Read the model definition and answer for the solid it produces. Units are mm, in the model's axes. A direction names the side the tool comes from. Coordinates: 2 decimals unless noted, no trailing zeros. Write each loop counter-clockwise with the first axis right and the second up, starting at its lowest first coordinate (ties: lowest second). Pieces come first, ordered by that corner, then holes. Notation, with made-up numbers: (50.25, 36) -> (101.25, 36) arc R5 ccw to (101.25, 41) -> close; hole circle Ø1 at (81.5, 67). An arc over 180 degrees is marked (long way). One line per item, written item: value. Start each with the question number.
from build123d import *

# Parameters (mm, degrees)
BOSS_EXTRUDE1_DEPTH          = 6.604
SKETCH2_R                    = 3.175
BOSS_EXTRUDE2_DEPTH          = 4.572
SKETCH3_R                    = 1.7907
CUT_EXTRUDE1_DEPTH           = 30.055416707
SKETCH4_R                    = 2.0193
CUT_EXTRUDE2_DEPTH           = 26.214451888
CUT_EXTRUDE2_DRAFT           = -4
CUT_EXTRUDE2_PROFILE_2_DEPTH = 26.214451888
CUT_EXTRUDE2_PROFILE_2_DRAFT = -4
SKETCH5_R                    = 1.7907
CUT_EXTRUDE3_DEPTH           = 6.604
SKETCH6_R                    = 2.0193
CUT_EXTRUDE4_DEPTH           = 6.604
CUT_EXTRUDE4_DRAFT           = -4
CUT_EXTRUDE4_PROFILE_2_DEPTH = 6.604
CUT_EXTRUDE4_PROFILE_2_DRAFT = -4


with BuildPart() as part:
    # Sketch1 → Boss-Extrude1 (new body)
    with BuildSketch(Plane.XY):
        Polygon((-11.5, -6.25), (-11.5, 6.25), (11.5, 6.25), (11.5, -6.25), (11.5, -9.498), (19.05, -9.498), (19.05, -6.25), (19.05, 10.822), (-19.05, 10.822), (-19.05, -6.25), (-19.05, -9.498), (-11.5, -9.498), align=None)
    extrude(amount=BOSS_EXTRUDE1_DEPTH)

    # Sketch2 → Boss-Extrude2 (add)
    with BuildSketch(Plane(origin=(0, 10.822, 0), x_dir=(1, 0, 0), z_dir=(0, 1, 0))):
        with BuildLine():
            Line((2.08, -11.464), (2.08, -6.604))
            Line((2.08, -6.604), (17.32, -6.604))
            Line((17.32, -6.604), (17.32, -11.464))
            ThreePointArc((17.32, -11.464), (9.7, -19.084), (2.08, -11.464))
        make_face()
        with Locations(Location((9.7, -11.464, 0), (0, 0, 180))):
            Circle(SKETCH2_R, mode=Mode.SUBTRACT)
    extrude(amount=-BOSS_EXTRUDE2_DEPTH)

    # Sketch3 → Cut-Extrude1 (cut, through all)
    with BuildSketch(Plane(origin=(0, 0, 0), x_dir=(-1, 0, 0), z_dir=(0, 0, -1))):
        with Locations((13.9, 0)):
            Circle(SKETCH3_R)
        with Locations((-13.9, 0)):
            Circle(SKETCH3_R)
    extrude(amount=-CUT_EXTRUDE1_DEPTH, mode=Mode.SUBTRACT)


with BuildPart() as cut_extrude2_tool:
    # Sketch4 → Cut-Extrude2 (with draft: the straight prism first)
    with BuildSketch(Plane.XY.offset(6.604)):
        with Locations((-13.9, 0)):
            Circle(SKETCH4_R)
    extrude(amount=-CUT_EXTRUDE2_DEPTH)
    # Cut-Extrude2: the draft: its side faces are tilted about the plane it starts from
    cut_extrude2_sides = [cut_extrude2_tool.faces().sort_by_distance(p)[0] for p in [
        (-15.9193, 0, -6.503225944),
    ]]
    draft(cut_extrude2_sides, Plane.XY.offset(6.604), CUT_EXTRUDE2_DRAFT)


with BuildPart() as part_1:
    add(part.part)

    # Cut-Extrude2: cut by cut_extrude2_tool
    add(cut_extrude2_tool.part, mode=Mode.SUBTRACT)


with BuildPart() as cut_extrude2_profile_2_tool:
    # Sketch4 → Cut-Extrude2 profile 2 (with draft: the straight prism first)
    with BuildSketch(Plane.XY.offset(6.604)):
        with Locations((13.9, 0)):
            Circle(SKETCH4_R)
    extrude(amount=-CUT_EXTRUDE2_PROFILE_2_DEPTH)
    # Cut-Extrude2 profile 2: the draft: its side faces are tilted about the plane it starts from
    cut_extrude2_profile_2_sides = [cut_extrude2_profile_2_tool.faces().sort_by_distance(p)[0] for p in [
        (11.8807, 0, -6.503225944),
    ]]
    draft(cut_extrude2_profile_2_sides, Plane.XY.offset(6.604), CUT_EXTRUDE2_PROFILE_2_DRAFT)


with BuildPart() as part_2:
    add(part_1.part)

    # Cut-Extrude2 profile 2: cut by cut_extrude2_profile_2_tool
    add(cut_extrude2_profile_2_tool.part, mode=Mode.SUBTRACT)

    # Sketch5 → Cut-Extrude3 (cut)
    with BuildSketch(Plane(origin=(19.05, 0, 0), x_dir=(0, 0, -1), z_dir=(1, 0, 0))):
        with Locations(Location((-3.302, 7.647, 0), (0, 0, 90))):
            Circle(SKETCH5_R)
        with Locations(Location((-3.302, -6.323, 0), (0, 0, 90))):
            Circle(SKETCH5_R)
    extrude(amount=-CUT_EXTRUDE3_DEPTH, mode=Mode.SUBTRACT)


with BuildPart() as cut_extrude4_tool:
    # Sketch6 → Cut-Extrude4 (with draft: the straight prism first)
    with BuildSketch(Plane(origin=(19.05, 0, 0), x_dir=(0, 0, -1), z_dir=(1, 0, 0))):
        with Locations((-3.302, 7.647)):
            Circle(SKETCH6_R)
    extrude(amount=-CUT_EXTRUDE4_DEPTH)
    # Cut-Extrude4: the draft: its side faces are tilted about the plane it starts from
    cut_extrude4_sides = [cut_extrude4_tool.faces().sort_by_distance(p)[0] for p in [
        (15.748, 7.647, 5.3213),
    ]]
    draft(cut_extrude4_sides, Plane(origin=(19.05, 0, 0), x_dir=(0, 0, -1), z_dir=(1, 0, 0)), CUT_EXTRUDE4_DRAFT)


with BuildPart() as part_3:
    add(part_2.part)

    # Cut-Extrude4: cut by cut_extrude4_tool
    add(cut_extrude4_tool.part, mode=Mode.SUBTRACT)


with BuildPart() as cut_extrude4_profile_2_tool:
    # Sketch6 → Cut-Extrude4 profile 2 (with draft: the straight prism first)
    with BuildSketch(Plane(origin=(19.05, 0, 0), x_dir=(0, 0, -1), z_dir=(1, 0, 0))):
        with Locations((-3.302, -6.323)):
            Circle(SKETCH6_R)
    extrude(amount=-CUT_EXTRUDE4_PROFILE_2_DEPTH)
    # Cut-Extrude4 profile 2: the draft: its side faces are tilted about the plane it starts from
    cut_extrude4_profile_2_sides = [cut_extrude4_profile_2_tool.faces().sort_by_distance(p)[0] for p in [
        (15.748, -6.323, 5.3213),
    ]]
    draft(cut_extrude4_profile_2_sides, Plane(origin=(19.05, 0, 0), x_dir=(0, 0, -1), z_dir=(1, 0, 0)), CUT_EXTRUDE4_PROFILE_2_DRAFT)


with BuildPart() as part_4:
    add(part_3.part)

    # Cut-Extrude4 profile 2: cut by cut_extrude4_profile_2_tool
    add(cut_extrude4_profile_2_tool.part, mode=Mode.SUBTRACT)


solid = part_4.part
1. A cutting plane is placed at A-A on y = 0. Give the vertices of the cut face in (x, z), then the cut area to 3 significant figures.
2. For a pull along Y with two mould halves and no side action, classify faces 1 (the face through (-11.5, -2, 3)), 2 (the face through (12.446, 8, 3)), 3 (the face through (-15, -9.498, 3)) as +Y half, -Y half, draft (parallel to the pull), parting line (faces both ways), or undercut.
3. Given pin 1 (3 mm diameter, centred on x = 13.9, y = 0, fed in from -Z); pin 2 (2.5 mm diameter, centred on y = 8, z = 9, fed in from +X); pin 3 (1.4 mm diameter, centred on y = 9.5, z = 8.5, fed in from -X); pin 4 (8.5 mm diameter, centred on x = 17, y = -2, fed in from +Z), each flat-ended and moving along its own axis, determine where each tip first touches the part or whether it passes through.
4. Find the intervals of material crossed by probe 1 along X at (y, z) = (0, 1.5); probe 2 along X at (y, z) = (-3.25, 3.25); probe 3 along Y at (x, z) = (13.9, 1.05), in increasing order. Write a range as from..to.
5. A cutting plane is placed at C-C on y = -3.25. Give the vertices of the cut face in (x, z), then the cut area to 3 significant figures.
6. A cutting plane is placed at D-D on x = 13.9. Give the vertices of the cut face in (y, z).
7. A cutting plane is placed at B-B on x = -13.9. Give the vertices of the cut face in (y, z), then the cut area to 3 significant figures.
8. A tool of negligible diameter and unlimited length cuts with its end or side. For faces 4 (the face through (12.246, -0.686, 1.644)), 5 (the face through (6, 6.25, 7)), 6 (the face through (17.32, 9, 9)), 7 (the face through (14.14, -5.5, 1.71)), 8 (the face through (5, 10.822, 7)), from which of +Z, -Z, +X, -X, +Y, -Y can it reach the whole face along a straight path? Write none if from no direction.
Derived:
1. outline: (-19.05, 0) -> (-15.69, 0) -> (-15.69, 3.33) -> (-15.92, 6.6) -> (-19.05, 6.6) -> close; (-12.11, 0) -> (-11.5, 0) -> (-11.5, 6.6) -> (-11.88, 6.6) -> (-12.11, 3.33) -> close; (11.5, 0) -> (12.11, 0) -> (12.11, 3.33) -> (11.88, 6.6) -> (11.5, 6.6) -> close; (15.69, 0) -> (19.05, 0) -> (19.05, 6.6) -> (15.92, 6.6) -> (15.69, 3.33) -> close
1. area: 50.9 mm2
2. face 1: draft
2. face 2: undercut
2. face 3: -Y half
3. pin 1: passes through
3. pin 2: stops at x = 17.32
3. pin 3: stops at x = 2.08
3. pin 4: stops at z = 6.6
4. probe 1: x = -19.05..-15.69, -12.11..-11.5, 11.5..12.11, 15.69..19.05
4. probe 2: x = -19.05..-11.5, 11.5..19.05
4. probe 3: y = -9.5..-1.79, 1.79..10.82
5. outline: (-19.05, 0) -> (-11.5, 0) -> (-11.5, 6.6) -> (-19.05, 6.6) -> close; (11.5, 0) -> (19.05, 0) -> (19.05, 6.6) -> (11.5, 6.6) -> close
5. area: 99.7 mm2
6. outline: (-9.5, 0) -> (-1.79, 0) -> (-1.79, 3.33) -> (-2.02, 6.6) -> (-9.5, 6.6) -> close; (1.79, 0) -> (10.82, 0) -> (10.82, 17.82) -> (6.25, 17.82) -> (6.25, 6.6) -> (2.02, 6.6) -> (1.79, 3.33) -> close; hole circle Ø3.58 at (-6.32, 3.3); hole circle Ø3.58 at (7.65, 3.3)
7. outline: (-9.5, 0) -> (-1.79, 0) -> (-1.79, 3.33) -> (-2.02, 6.6) -> (-9.5, 6.6) -> close; (1.79, 0) -> (10.82, 0) -> (10.82, 6.6) -> (2.02, 6.6) -> (1.79, 3.33) -> close
7. area: 110 mm2
8. face 4: +Z, -Z
8. face 5: +Z, -Y
8. face 6: +Z, +X, +Y, -Y
8. face 7: +X
8. face 8: +Z, -Z, +X, -X, +Y
